Could you check a few things on this model? Use its own coordinates, in mm. A direction names the side the tool comes from. Give positions to 0.01 mm unless a question says otherwise; leave off trailing zeros. Loops run counter-clockwise (first coordinate to the right, second up) from the corner with the lowest first, then second, coordinate; pieces in that order, holes last.
1. Thinking about a two-plate mould opening in X: for faces 3 (the flat face through (-1, 1, 0)), 4 (the flat face through (-1, 1, 4)), 5 (the flat face through (64.978, -1, 3)), 6 (the cylindrical face through (51.14, -44.58, 5.01)), which applies, +X half, -X half, draft (parallel to the pull), parting line (faces both ways), or undercut?
2. For P1, Ø3, axis at x = 32.5, y = 21.5, coming from the +Z side, with a flat end and sliding along its axis, tell me the tip position at first contact or that it passes through.
3. Imagine slicing it at A-A (y = -18). List the corners of the cut face in (x, z) for me, plus the area to 3 significant figures.
4. I need wall thicknesses on line 1 along X through (y, z) = (-48.5, 0.65); line 2 along Y through (x, z) = (-23, 4.95); line 3 along X through (y, z) = (38, 4.25). Which ranges of each line are inside material? Lowest first, please.
5. For faces 1 (the cylindrical face through (-51.455, 44.07, 5.014)), 2 (the cylindrical face through (-60.92, 60.49, 2.96)), which set-ups out of +Z, -Z, +X, -X, +Y, -Y let a thin tool reach every point of the face, with its end or its side?
6. Imagine slicing it at B-B (x = 5). List the corners of the cut face in (y, z) for me.
Autodesk Inventor part; units mm, degrees
ref_plane "YZ Plane" through (0, 0, 0) normal (1, 0, 0) x (0, 1, 0)
ref_plane "XZ Plane" through (0, 0, 0) normal (0, 1, 0) x (-1, 0, 0)
ref_plane "XY Plane" through (0, 0, 0) normal (0, 0, 1) x (1, 0, 0)
sketch "Esboço1" plane through (0, 0, 0) normal (0, 0, 1) x (1, 0, 0)
  line L0 (60.7325, -52.1672) -> (60.7325, 51.7628)
  line L1 (-60.7775, 51.7628) -> (-60.7775, -52.1672)
  line L2 (60.7325, -0.2022) -> (-60.7775, -0.2022)
  line L3 (64.9775, 67.2978) -> (-65.0225, 67.2978)
  line L4 (-65.0225, 67.2978) -> (-65.0225, -67.7022)
  line L5 (-65.0225, -67.7022) -> (64.9775, -67.7022)
  line L6 (64.9775, -67.7022) -> (64.9775, 67.2978)
  line L7 (64.9775, 67.2978) -> (-65.0225, -67.7022) construction
  line L8 (-65.0225, 67.2978) -> (64.9775, -67.7022) construction
  circle A0 centre (55.9625, -48.1472) radius 1.8
  circle A1 centre (55.9625, 47.3828) radius 1.8
  circle A2 centre (-56.4575, 47.3828) radius 1.8
  circle A3 centre (-56.4575, -48.1472) radius 1.8
  circle A4 centre (-56.4575, 47.3828) radius 0.7501
  circle A5 centre (-56.4575, -48.1472) radius 1.059
  circle A6 centre (55.9625, -48.1472) radius 0.7793
  circle A7 centre (55.9625, 47.3828) radius 0.9848
  point P0 (0, 0)
  point P1 (-0.0225, -0.2022)
  dimension "d0" = 135
  dimension "d1" = 130
extrude "Extrusão1" add sketch "Esboço1" along normal blind 6 contours L6 L5 L4 L3 | A0 | A1 | A2 | A3
sketch "Esboço2" plane through (0, 0, 6) normal (0, 0, 1) x (1, 0, 0)
  circle A0 centre (-56.4575, 47.3828) radius 0.7501
  circle A1 centre (55.9625, 47.3828) radius 0.9848
  circle A2 centre (55.9625, -48.1472) radius 0.7793
  circle A3 centre (-56.4575, -48.1472) radius 1.059
  point P0 (0, 0)
hole "Furo1" at (-56.4575, 47.3828, 6) at (55.9625, 47.3828, 6) at (55.9625, -48.1472, 6) at (-56.4575, -48.1472, 6) direction (0, 0, -1) diameter 2.459 end through all
sketch "Esboço3" plane through (0, 0, 6) normal (0, 0, 1) x (1, 0, 0)
  line L0 (64.9775, 67.2978) -> (-65.0225, 67.2978)
  line L1 (-0.0225, 67.2978) -> (-0.0225, -67.7022)
  line L2 (-65.0225, -67.7022) -> (64.9775, -67.7022)
  line L3 (-58.0225, -52.7022) -> (57.9775, -52.7022)
  line L4 (57.9775, -52.7022) -> (57.9775, 52.2978)
  line L5 (57.9775, 52.2978) -> (-58.0225, 52.2978)
  line L6 (-58.0225, 52.2978) -> (-58.0225, -52.7022)
  line L7 (-58.0225, -52.7022) -> (57.9775, 52.2978) construction
  line L8 (57.9775, -52.7022) -> (-58.0225, 52.2978) construction
  circle A0 centre (-56.4575, 47.3828) radius 1.2295
  circle A1 centre (-56.4575, 47.3828) radius 6
  circle A2 centre (55.9625, 47.3828) radius 1.2295
  circle A3 centre (55.9625, 47.3828) radius 6
  circle A4 centre (-56.4575, -48.1472) radius 1.2295
  circle A5 centre (-56.4575, -48.1472) radius 6
  circle A6 centre (55.9625, -48.1472) radius 1.2295
  circle A7 centre (55.9625, -48.1472) radius 6
  point P0 (-0.0225, -0.2022)
  point P1 (-58.0225, -42.3549)
  point P2 (-52.5521, -52.7022)
  point P3 (52.0572, -52.7022)
  point P4 (57.9775, -42.4957)
  point P5 (57.9775, 41.7313)
  point P6 (52.5212, 52.2978)
  point P7 (-53.0161, 52.2978)
  point P8 (-58.0225, 41.5905)
  dimension "d16" = 116
  dimension "d17" = 105
  dimension "d18" = 12
extrude "Extrusão2" cut sketch "Esboço3" against normal blind 2 contours L5 A3 L4 A7 L3 L1 | L1 L3 A5 L6 A1 L5
fillet "Arredondamento1" radius 2 8 edges at (-58.0225, -42.3549, 5) (-52.5521, -52.7022, 5) (52.0572, -52.7022, 5) (57.9775, -42.4957, 5) (57.9775, 41.7313, 5) (52.5212, 52.2978, 5) (-53.0161, 52.2978, 5) (-58.0225, 41.5905, 5)
sketch "Esboço4" plane through (0, 0, 6) normal (0, 0, 1) x (1, 0, 0)
  line L0 (0, 0) -> (0, -87.1961)
  line L1 (0, 0) -> (-82.4398, 0)
  line L2 (-65.0225, -67.7022) -> (64.9775, -67.7022)
  line L3 (-65.0225, 67.2978) -> (-65.0225, -67.7022)
  line L4 (-65.0225, 67.7022) -> (64.9775, 67.7022)
  point P0 (-59.0225, -61.7022)
  point P1 (59.0225, -61.7022)
  point P2 (65.0225, -67.7022)
  point P3 (-59.0225, 61.7022)
  point P4 (65.0225, 67.7022)
  point P5 (59.0225, 61.7022)
  dimension "d22" = 6
  dimension "d23" = 6
hole "Furo2" at (-59.0225, -61.7022, 6) at (59.0225, -61.7022, 6) at (59.0225, 61.7022, 6) at (-59.0225, 61.7022, 6) direction (0, 0, -1) diameter 4.5 end through all
fillet "Arredondamento2" radius 2 4 edges at (64.9775, -67.7022, 3) (-65.0225, -67.7022, 3) (-65.0225, 67.2978, 3) (64.9775, 67.2978, 3)
properties part number "chapa da pcb"
Derived:
1. face 3: draft
1. face 4: undercut
1. face 5: +X half
1. face 6: undercut
2. P1: stops at z = 4
3. outline: (-65.02, 0) - (64.98, 0) - (64.98, 6) - (57.98, 6) - (57.98, 4) - (-58.02, 4) - (-58.02, 6) - (-65.02, 6) - close
3. area: 548 mm2
4. line 1: x = -65.02 to -57.64, -55.28 to 54.78, 57.14 to 64.98
4. line 2: y = -67.7 to -52.7, 52.3 to 67.3
4. line 3: x = -65.02 to -58.02, 57.98 to 64.98
5. face 1: +Z
5. face 2: +Z, -Z
6. outline: (-67.7, 0) - (67.3, 0) - (67.3, 6) - (52.3, 6) - (52.3, 4) - (-52.7, 4) - (-52.7, 6) - (-67.7, 6) - close
